Print and shaded views of the part. All mm, measured from the part's lowest x, y and z. A direction names the side the tool comes from. Round coordinates to 2 decimals unless told otherwise and drop trailing zeros. Loops run counter-clockwise (first coordinate to the right, second up) from the corner with the lowest first, then second, coordinate; pieces in that order, holes last. Notation, with made-up numbers: (42, 12) - (61, 12) arc R25 cw to (61, 47) - close; hole circle Ø2 at (76, 56.5). An arc over 180 degrees is marked (long way). Answer as a JSON object with one key per item and string values.
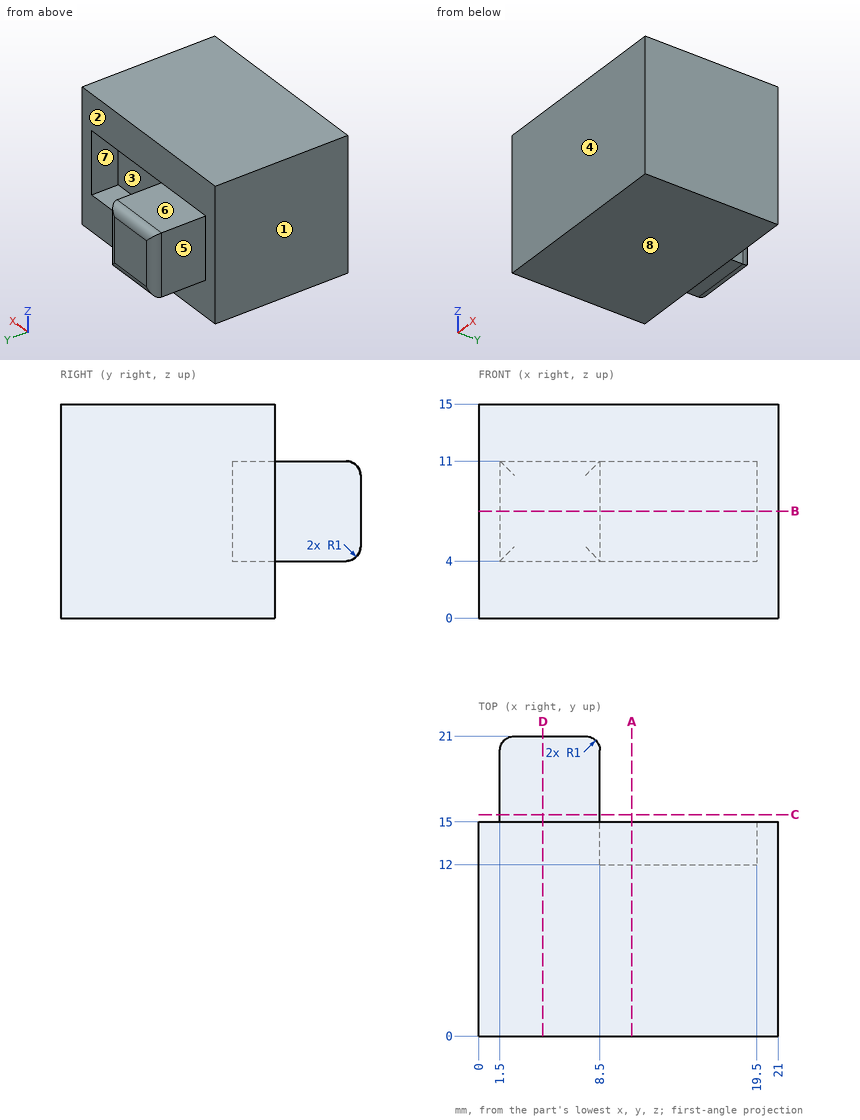
1) Probe probe 1 along X at (y, z) = (12.25, 6.75); probe 2 along Z at (x, y) = (18.5, 14); probe 3 along X at (y, z) = (16, 10.5). List the from-to ranges inside material, lowest first.
Values follow:
{"probe 1": "0 to 8.5, 19.5 to 21", "probe 2": "0 to 4, 11 to 15", "probe 3": "1.5 to 8.5"}
2) Drop flat-ended pins along their axis: P1, Ø1.5, axis at x = 6, y = 18.5, coming from the -Z side; P2, Ø5.5, axis at x = 6, y = 18, coming from the +Z side; P3, Ø3.5, axis at y = 17.5, z = 8.5, coming from the +X side. Give the stop position or say it passes through.
Values follow:
{"P1": "z = 4", "P2": "z = 11", "P3": "x = 8.5"}
3) Two-plate mould, pull along X, no slides. Class the marked faces 1, 2 and 3: pulls with the +X half, pulls with the -X half, needs draft (parallel to the pull), parting line crosses it, or undercut.
Values follow:
{"face 1": "pulls with the -X half", "face 2": "needs draft", "face 3": "undercut"}
4) Slice it at B-B on z = 7.5. List the corners of the cut face in (x, y), then the cut area to 3 significant figures.
Values follow:
{"outline": "(0, 0) - (21, 0) - (21, 15) - (19.5, 15) - (19.5, 12) - (8.5, 12) - (8.5, 20) arc R1 ccw to (7.5, 21) - (2.5, 21) arc R1 ccw to (1.5, 20) - (1.5, 15) - (0, 15) - close", "area": "324 mm²"}
5) Slice it at D-D on x = 4.5. List the corners of the cut face in (y, z), then the cut area to 3 significant figures.
Values follow:
{"outline": "(0, 0) - (15, 0) - (15, 4) - (20, 4) arc R1 ccw to (21, 5) - (21, 10) arc R1 ccw to (20, 11) - (15, 11) - (15, 15) - (0, 15) - close", "area": "267 mm²"}
6) Tool access for the marked faces 4, 5, 6, 7 and 8: list every direction of +Z, -Z, +X, -X, +Y, -Y with a clear straight run to the whole face (end or side of a thin tool).
Values follow:
{"face 4": "+Z, -Z, +X, -X, -Y", "face 5": "+Z, -Z, -X, +Y", "face 6": "+Z, +X, -X, +Y", "face 7": "+Y", "face 8": "-Z, +X, -X, +Y, -Y"}
7) Slice it at C-C on y = 15.5. List the corners of the cut face in (x, z).
Values follow:
{"outline": "(1.5, 4) - (8.5, 4) - (8.5, 11) - (1.5, 11) - close"}
8) Slice it at A-A on x = 10.75. List the corners of the cut face in (y, z), then the cut area to 3 significant figures.
Values follow:
{"outline": "(0, 0) - (15, 0) - (15, 4) - (12, 4) - (12, 11) - (15, 11) - (15, 15) - (0, 15) - close", "area": "204 mm²"}
